The model under review builds one solid part; all positions refer to its coordinate system, in mm. Face numbers are marked on the shaded views. A direction names the side the tool comes from. Round coordinates to 2 decimals unless told otherwise and drop trailing zeros. Loops run counter-clockwise (first coordinate to the right, second up) from the corner with the lowest first, then second, coordinate; pieces in that order, holes last. Notation, with made-up numbers: (-38, 15) -> (-1, 15) arc R22 cw to (-1, 50) -> close; hole circle Ø3 at (-28, 2). An arc over 180 degrees is marked (long way). Return JSON: item names as keys, results as strings. Group by question number.
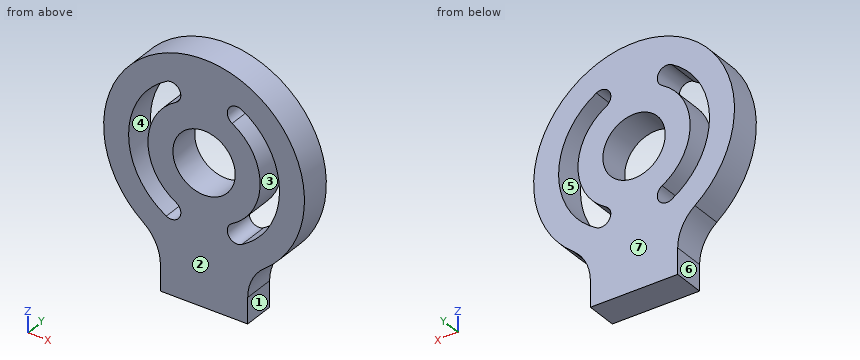
```python
from build123d import *

# Parameters (mm, degrees)
SKETCH001_AS_DRAWN_R                 = 5
EXTRUDE001_DEPTH                     = 5
EXTRUDE001_ONTO_SKETCH001_ROLL_ANGLE = 90
FILLET_R                             = 7


with BuildPart() as part:
    # Sketch001 as drawn → Extrude001 (new)
    with BuildSketch(Plane.XY):
        with BuildLine():
            Line((-7, 0), (7, 0))
            Line((7, 0), (7, 8))
            ThreePointArc((7, 8), (0, 38.598621), (-7, 8))
            Line((-7, 0), (-7, 8))
        make_face()
        with Locations((0, 22.498621)):
            Circle(SKETCH001_AS_DRAWN_R, mode=Mode.SUBTRACT)
        with BuildLine():
            ThreePointArc((-6.05, 32.977528), (-12.1, 22.498621), (-6.05, 12.019713))
            ThreePointArc((-6.05, 12.019713), (-3.932661, 12.587053), (-4.5, 14.704392))
            ThreePointArc((-4.5, 30.292849), (-9, 22.498621), (-4.5, 14.704392))
            ThreePointArc((-4.5, 30.292849), (-3.932661, 32.410189), (-6.05, 32.977528))
        make_face(mode=Mode.SUBTRACT)
        with BuildLine():
            ThreePointArc((4.5, 14.704392), (9, 22.498621), (4.5, 30.292849))
            ThreePointArc((6.05, 32.977528), (3.932661, 32.410189), (4.5, 30.292849))
            ThreePointArc((6.05, 12.019713), (12.1, 22.498621), (6.05, 32.977528))
            ThreePointArc((4.5, 14.704392), (3.932661, 12.587053), (6.05, 12.019713))
        make_face(mode=Mode.SUBTRACT)
    extrude(amount=-EXTRUDE001_DEPTH)


with BuildPart() as part_1:
    # Extrude001 onto Sketch001 roll: moved
    add(part.part.rotate(Axis((0, 0, 0), (1, 0, 0)), EXTRUDE001_ONTO_SKETCH001_ROLL_ANGLE))


with BuildPart() as part_2:
    # Extrude001 onto Sketch001 placement: moved
    add(part_1.part)

    # Fillet
    fillet_edges = [part_2.edges().sort_by_distance(p)[0] for p in [
        (7, 2.5, 8),
        (-7, 2.5, 8),
    ]]
    fillet(fillet_edges, radius=FILLET_R)


solid = part_2.part
```
1. We need section B-B, the plane z = 16. Write out the cut boundary in (x, y).
2. Tool access review of the marked faces 5, 6 and 7: name each direction out of +Z, -Z, +X, -X, +Y, -Y from which nothing blocks a thin tool from reaching the whole face with its end or side.
3. We need section A-A, the plane x = 0. Write out the cut boundary in (y, z), then the cut area to 3 significant figures.
4. We need section D-D, the plane x = -8.5. Write out the cut boundary in (y, z), then the cut area to 3 significant figures.
5. Wall thickness on line 1 (X direction, y = 2.9, z = 25.5); line 2 (X direction, y = 3.25, z = 12); line 3 (Z direction, x = 0, y = 1.15): over which ranges is each line inside the solid? List them lowest first.
6. For P1, Ø1.5, axis at y = 3.5, z = 14, coming from the -X side; P2, Ø1.2, axis at y = 2.5, z = 2.5, coming from the -X side; P3, Ø1.5, axis at y = 1.5, z = 32.5, coming from the +X side, all flat-tipped, find the tip position at first contact; note any pin that passes through.
7. We need section C-C, the plane y = 1.85. Write out the cut boundary in (x, z) (3 decimals), then the cut area to 3 significant figures.
8. Draft analysis for pull direction X (two halves, no side actions). For the marked faces 1, 2, 3 and 4, state which applies: pulls with the +X half, pulls with the -X half, needs draft (parallel to the pull), parting line crosses it, or undercut.
Check sheet entries:
{
 "1": {"outline": "(-14.73, 0) -> (-10.21, 0) -> (-10.21, 5) -> (-14.73, 5) -> close; (-6.23, 0) -> (6.23, 0) -> (6.23, 5) -> (-6.23, 5) -> close; (10.21, 0) -> (14.73, 0) -> (14.73, 5) -> (10.21, 5) -> close"},
 "2": {"face 5": "+Y, -Y", "face 6": "-Z, -X, +Y, -Y", "face 7": "+Z, -Z, +X, -X, +Y"},
 "3": {"outline": "(0, 0) -> (5, 0) -> (5, 17.5) -> (0, 17.5) -> close; (0, 27.5) -> (5, 27.5) -> (5, 38.6) -> (0, 38.6) -> close", "area": "143 mm²"},
 "4": {"outline": "(0, 8.45) -> (5, 8.45) -> (5, 13.89) -> (0, 13.89) -> close; (0, 19.54) -> (5, 19.54) -> (5, 25.46) -> (0, 25.46) -> close; (0, 31.11) -> (5, 31.11) -> (5, 36.17) -> (0, 36.17) -> close", "area": "82.1 mm²"},
 "5": {"line 1": "x = -15.82 to -11.72, -8.48 to -4, 4 to 8.48, 11.72 to 15.82", "line 2": "x = -12.21 to -6.01, -4.54 to 4.54, 6.01 to 12.21", "line 3": "z = 0 to 17.5, 27.5 to 38.6"},
 "6": {"P1": "stops at x = -14.11", "P2": "stops at x = -7", "P3": "stops at x = 13.18"},
 "7": {"outline": "(-9.758, 9.692) arc R7 cw to (-7, 4.124) -> (-7, 0) -> (7, 0) -> (7, 4.124) arc R7 cw to (9.758, 9.692) arc R16.1 ccw (long way) to start; hole (-6.05, 12.02) arc R1.55 ccw to (-4.5, 14.704) arc R9 cw to (-4.5, 30.293) arc R1.55 ccw to (-6.05, 32.978) arc R12.1 ccw to start; hole circle Ø10 at (0, 22.499); hole (4.5, 14.704) arc R1.55 ccw to (6.05, 12.02) arc R12.1 ccw to (6.05, 32.978) arc R1.55 ccw to (4.5, 30.293) arc R9 cw to start", "area": "685 mm²"},
 "8": {"face 1": "pulls with the +X half", "face 2": "needs draft", "face 3": "undercut", "face 4": "undercut"}
}
